Input: part model. Units: mm. Frame: model coordinates. Round coordinates to 2 decimals unless told otherwise and drop trailing zeros. Loops run counter-clockwise (first coordinate to the right, second up) from the corner with the lowest first, then second, coordinate; pieces in that order, holes last. Notation, with made-up numbers: M 8,24.25 L 48,24.25 A28 ccw 48,46.25 Z; hole C 49.5,-25.5 d10. An arc over 180 degrees is marked long. Return JSON: item names as keys, results as strings. Group by question number.
1) Mould query, pull axis Z, two halves, no side actions, for faces 1 (the face through (-0.129, 1.132, -2.948)), 2 (the face through (-0.08, -8.3, -1.94)), 3 (the face through (1, -23.05, -2)). Classes: +Z half, -Z half, draft (parallel to the pull), parting line (faces both ways), or undercut.
2) Section A-A (y = -16.5). Output: boundary loops of the cut face in (x, z), plus the area to 3 significant figures.
3) Contact query for flat-ended pins moving along their axis: P1, Ø1.4, axis at y = 11.5, z = 3, coming from the -X side; P2, Ø3.5, axis at x = 0, z = 0, coming from the -Y side; P3, Ø3, axis at y = -9, z = -1.5, coming from the -X side; P4, Ø1.5, axis at y = 4, z = 0.5, coming from the +X side. Output: stop coordinate, or through.
4) Material intervals for line 1 (X direction, y = -17, z = 0); line 2 (Z direction, x = 1.5, y = -13); line 3 (Y direction, x = 1, z = -2.5), sorted ascending. Write a range as from..to.
from build123d import *

# Parameters (mm, degrees)
CUT_EXTRUDE1_DEPTH      = 27.518252873
CUT_EXTRUDE1_DEPTH_BACK = 27.518252873
SKETCH4_W               = 0.127
SKETCH4_H               = 4.445496727
CHAMFER1_SIZE           = 1.016
CHAMFER1_SIZE2          = 0.088888482
FILLET1_R               = 0.254


with BuildPart() as part:
    # Sketch3 → Revolve1 (revolve)
    with BuildSketch(Plane(origin=(0, 0, 0), x_dir=(0, 0, -1), z_dir=(1, 0, 0)), mode=Mode.PRIVATE) as revolve1_sk:
        with BuildLine():
            Line((1.9431, -9.0805), (1.9431, 6.045643841))
            add(Edge.make_bspline(
                [(1.9431, 6.045643841), (1.9431, 10.091751432), (1.891096799, 23.164078911), (1.955698004, 25.891289644), (2.657297247, 26.530501845), (3.65125, 25.2095)],
                knots=[0, 0, 0, 0, 0.515431556, 0.615431556, 1, 1, 1, 1], degree=3))
            Line((3.65125, 25.2095), (3.20458454, 25.2095))
            ThreePointArc((3.20458454, 25.2095), (3.024979417, 25.135105122), (2.95058454, 24.9555))
            Line((2.95058454, 24.9555), (2.95058454, 24.211681499))
            Line((2.95058454, 24.211681499), (2.95058454, -9.0805))
            Line((2.95058454, -9.0805), (2.95058454, -23.0505))
            Line((2.95058454, -23.0505), (1.9431, -23.0505))
            Line((1.9431, -23.0505), (1.9431, -9.0805))
        make_face()
    revolve(revolve1_sk.sketch.rotate(Axis((0, 25.2095, 0), (0, -1, 0)), 180), axis=Axis((0, 25.2095, 0), (0, -1, 0)))

    # Sketch4 → Cut-Extrude1 (cut, two sides: drawn at the far end of the back side and taken through both)
    with BuildSketch(Plane(origin=(0, 0, 0), x_dir=(1, 0, 0), z_dir=(0, 1, 0)).offset(-CUT_EXTRUDE1_DEPTH_BACK)):
        with Locations((0, -2.222748364)):
            Rectangle(SKETCH4_W, SKETCH4_H)
    extrude(amount=CUT_EXTRUDE1_DEPTH + CUT_EXTRUDE1_DEPTH_BACK, mode=Mode.SUBTRACT)

    # Chamfer1
    chamfer1_edges = [part.edges().sort_by_distance(p)[0] for p in [
        (0, -23.0505, -2.95058454),
    ]]
    chamfer1_side = [part.faces().sort_by_distance(p)[0] for p in [
        (0, 0.9525, -2.95058454),
    ]]
    chamfer(chamfer1_edges, length=CHAMFER1_SIZE, length2=CHAMFER1_SIZE2, reference=chamfer1_side[0])

    # Fillet1
    fillet1_edges = [part.edges().sort_by_distance(p)[0] for p in [
        (0, -23.0505, -2.861696057),
    ]]
    fillet(fillet1_edges, radius=FILLET1_R)


solid = part.part
Returned:
{
 "1": {"face 1": "parting line", "face 2": "undercut", "face 3": "draft"},
 "2": {"outline": "M -0.06,1.94 L -0.06,2.95 A2.95 ccw long 0.06,2.95 L 0.06,1.94 A1.94 cw long Z", "area": "15.4 mm^2"},
 "3": {"P1": "stops at x = -1.85", "P2": "passes through", "P3": "stops at x = -2.95", "P4": "stops at x = 2.95"},
 "4": {"line 1": "x = -2.95..-1.94, 1.94..2.95", "line 2": "z = -2.54..-1.24, 1.24..2.54", "line 3": "y = -23.04..26"}
}
